```python
from build123d import *

# Parameters (mm, degrees)
SKETCH1_W                           = 17.4625
SKETCH1_H                           = 15.875
BOSS_EXTRUDE1_DEPTH                 = 9.525
SKETCH2_R                           = 4.365625
BOSS_EXTRUDE2_DEPTH                 = 4.7625
CUT_EXTRUDE1_START                  = -4.7625
CUT_EXTRUDE1_DEPTH                  = 4.7625
BOSS_EXTRUDE3_START                 = -0.0254
SKETCH4_R                           = 4.365625
BOSS_EXTRUDE3_DEPTH                 = 1.5875
CUT_EXTRUDE2_REACH                  = 28.553
CUT_EXTRUDE2_END_RADIUS             = 3
SKETCH6_W                           = 1.2375
SKETCH6_H                           = 6.35
CUT_EXTRUDE2_DIRECTION_2_REACH      = 28.553
CUT_EXTRUDE2_DIRECTION_2_END_RADIUS = 3
CHAMFER1_SIZE                       = 0.254
SKETCH7_W                           = 3.175
SKETCH7_H                           = 3.96875
BOSS_EXTRUDE4_DEPTH                 = 1.5875
BOSS_EXTRUDE5_DEPTH                 = 1.5875
FILLET1_R                           = 0.508


with BuildPart() as part:
    # Sketch1 → Boss-Extrude1 (new body)
    with BuildSketch(Plane(origin=(0, 0, 0), x_dir=(1, 0, 0), z_dir=(0, 1, 0))):
        Rectangle(SKETCH1_W, SKETCH1_H)
    extrude(amount=BOSS_EXTRUDE1_DEPTH)

    # Sketch2 → Boss-Extrude2 (add)
    with BuildSketch(Plane(origin=(0, 9.525, 0), x_dir=(1, 0, 0), z_dir=(0, 1, 0))):
        with Locations(Location((0, 0, 0), (0, 0, 90))):
            Circle(SKETCH2_R)
    extrude(amount=BOSS_EXTRUDE2_DEPTH)

    # Sketch3 → Cut-Extrude1 (cut)
    with BuildSketch(Plane(origin=(0, 14.2875, 0), x_dir=(1, 0, 0), z_dir=(0, 1, 0)).offset(CUT_EXTRUDE1_START)):
        with BuildLine():
            Line((-2.510057893, -3.571875), (2.510057893, -3.571875))
            ThreePointArc((2.510057893, -3.571875), (0, -4.365625), (-2.510057893, -3.571875))
        make_face()
        with BuildLine():
            Line((-2.510057893, 3.571875), (2.510057893, 3.571875))
            ThreePointArc((2.510057893, 3.571875), (0, 4.365625), (-2.510057893, 3.571875))
        make_face()
    extrude(amount=CUT_EXTRUDE1_DEPTH, mode=Mode.SUBTRACT)



with BuildPart() as body_2:
    # Sketch4 → Boss-Extrude3 (new body)
    with BuildSketch(Plane(origin=(0, 14.2875, 0), x_dir=(1, 0, 0), z_dir=(0, 1, 0)).offset(BOSS_EXTRUDE3_START)):
        Polygon((2.978766545, 5.159375), (-2.978766545, 5.159375), (-5.95753309, 0), (-2.978766545, -5.159375), (2.978766545, -5.159375), (5.95753309, 0), align=None)
        with Locations(Location((0, 0, 0), (0, 0, 270))):
            Circle(SKETCH4_R, mode=Mode.SUBTRACT)
    extrude(amount=-BOSS_EXTRUDE3_DEPTH)


with BuildPart() as part_1:
    add(part.part)

    add(body_2.part)  # Revolve1 merges body 2
    # Sketch5 → Revolve1 (revolve)
    with BuildSketch(Plane(origin=(0, 0, 0), x_dir=(0, 0, -1), z_dir=(1, 0, 0))):
        Polygon((-2.5, 14.2621), (-2.5, 15.2621), (-3, 15.2621), (-3, 23.7871), (0, 23.7871), (0, 14.2621), align=None)
    revolve(axis=Axis((0, 14.2621, 0), (0, -1, 0)))

    # Cut-Extrude2: up to this cylinder (the profile starts inside it)
    cut_extrude2_end = Plane(origin=(0, 20.6121, 0), z_dir=(0, 1, 0)) * Cylinder(CUT_EXTRUDE2_END_RADIUS, 64.106, mode=Mode.PRIVATE)
    # Sketch6 → Cut-Extrude2 (cut, up to the surface)
    with BuildSketch(Plane(origin=(0, 0, 0), x_dir=(0, 0, -1), z_dir=(1, 0, 0)), mode=Mode.PRIVATE) as cut_extrude2_sk1:
        with Locations((-2.38125, 20.6121)):
            Rectangle(SKETCH6_W, SKETCH6_H)
    cut_extrude2_tool1 = extrude(cut_extrude2_sk1.sketch, amount=-CUT_EXTRUDE2_REACH, mode=Mode.PRIVATE) & cut_extrude2_end
    add(cut_extrude2_tool1.solids().sort_by_distance((0, 20.6121, 2.38125))[0], mode=Mode.SUBTRACT)

    # Cut-Extrude2 direction 2: up to this cylinder (the profile starts inside it)
    cut_extrude2_direction_2_end = Plane(origin=(0, 20.6121, 0), z_dir=(0, 1, 0)) * Cylinder(CUT_EXTRUDE2_DIRECTION_2_END_RADIUS, 64.106, mode=Mode.PRIVATE)
    # Sketch6 → Cut-Extrude2 direction 2 (cut, up to the surface)
    with BuildSketch(Plane(origin=(0, 0, 0), x_dir=(0, 0, -1), z_dir=(1, 0, 0)), mode=Mode.PRIVATE) as cut_extrude2_direction_2_sk1:
        with Locations((-2.38125, 20.6121)):
            Rectangle(SKETCH6_W, SKETCH6_H)
    cut_extrude2_direction_2_tool1 = extrude(cut_extrude2_direction_2_sk1.sketch, amount=CUT_EXTRUDE2_DIRECTION_2_REACH, mode=Mode.PRIVATE) & cut_extrude2_direction_2_end
    add(cut_extrude2_direction_2_tool1.solids().sort_by_distance((0, 20.6121, 2.38125))[0], mode=Mode.SUBTRACT)

    # Chamfer1
    chamfer1_edges = [part_1.edges().sort_by_distance(p)[0] for p in [
        (0, 23.7871, -3),
    ]]
    chamfer(chamfer1_edges, length=CHAMFER1_SIZE)

    # Sketch7 → Boss-Extrude4 (add)
    with BuildSketch(Plane(origin=(0, 9.525, 0), x_dir=(1, 0, 0), z_dir=(0, 1, 0))):
        with Locations((10.31875, 0)):
            Rectangle(SKETCH7_W, SKETCH7_H)
    extrude(amount=-BOSS_EXTRUDE4_DEPTH)

    # Sketch8 → Boss-Extrude5 (add)
    with BuildSketch(Plane(origin=(0, 9.525, 0), x_dir=(1, 0, 0), z_dir=(0, 1, 0))):
        with BuildLine():
            Line((8.73125, 1.190625), (8.73125, -1.190625))
            ThreePointArc((8.73125, -1.190625), (9.921875, 0), (8.73125, 1.190625))
        make_face()
    extrude(amount=BOSS_EXTRUDE5_DEPTH)

    # Fillet1
    fillet1_edges = [part_1.edges().sort_by_distance(p)[0] for p in [
        (-8.73125, 9.525, 0),
        (0, 9.525, 7.9375),
        (8.73125, 9.525, 4.9609375),
        (0, 9.525, -7.9375),
        (8.73125, 4.7625, 7.9375),
        (-8.73125, 4.7625, 7.9375),
        (-8.73125, 4.7625, -7.9375),
        (8.73125, 4.7625, -7.9375),
        (8.73125, 9.525, -4.9609375),
        (8.73125, 8.73125, 1.984375),
        (8.73125, 8.73125, -1.984375),
        (11.90625, 8.73125, -1.984375),
        (11.90625, 8.73125, 1.984375),
        (10.31875, 9.525, 1.984375),
        (11.90625, 9.525, 0),
        (10.31875, 9.525, -1.984375),
    ]]
    fillet(fillet1_edges, radius=FILLET1_R)


solid = part_1.part
```
Work out the finished part from the listing and answer in its coordinate system (mm). A direction names the side the tool comes from. Coordinates: 2 decimals unless noted, no trailing zeros. Loops run counter-clockwise (first coordinate to the right, second up) from the corner with the lowest first, then second, coordinate; pieces in that order, holes last. Notation, with made-up numbers: M 42.25,-1 L 90.25,-1 A18 ccw 90.25,26 Z; hole C 35,28.5 d3. An arc over 180 degrees is marked long. Use CSV: the item, a comma, the result in double quotes. Start each with the question number.
(1) Given pin 1 Ø3 at (x, z) = (0.5, -0.5) entering from -Y; pin 2 Ø0.8 at (x, y) = (0, 13.5) entering from -Z; pin 3 Ø2.5 at (x, y) = (-0.5, 20.5) entering from +Z; pin 4 Ø10 at (x, y) = (2.5, 16) entering from +Z, each flat-ended and moving along its own axis, determine where each tip first touches the part or whether it passes through.
(2) Consider line 1 (Y direction, x = -3.25, z = -3.5) (3 decimals); line 2 (Y direction, x = 7.75, z = -5.75) (3 decimals); line 3 (X direction, y = 6, z = -1.75). Determine where each line is inside the solid, lowest interval first.
(3) Find section B-B, the plane z = -4.75. Give the vertices of the cut face in (x, y) (3 decimals), then the cut area to 3 significant figures.
(4) Find section D-D, the plane y = 5. Give the vertices of the cut face in (x, z).
(5) Find section A-A, the plane x = 0. State how many separate pieces and enclosed holes the cut face has, then the cut area to 3 significant figures.
(6) Find section C-C, the plane x = -7. Give the vertices of the cut face in (y, z) (1 decimal).
(7) For a pull along Z with two mould halves and no side action, classify faces 1 (the face through (11.906, 8.5, 0)), 2 (the face through (9.92, 10.31, 0.03)), 3 (the face through (0, 12, 3.572)) as +Z half, -Z half, draft (parallel to the pull), parting line (faces both ways), or undercut.
(8) For faces 4 (the face through (4.365, 11.078, 0.059)), 5 (the face through (0, 19, -3)), 6 (the face through (0, 21, 1.763)), 7 (the face through (4.49, 13.48, -2.54)), 8 (the face through (-4.447, 13.479, -2.616)), determine the directions among +Z, -Z, +X, -X, +Y, -Y from which every point of the face is accessible in a straight line to the end or side of a thin tool.
Recorded:
1,pin 1,"stops at y = 0"
1,pin 2,"stops at z = -5.16"
1,pin 3,"stops at z = 1.76"
1,pin 4,"stops at z = 5.16"
2,line 1,"y = 0 to 9.525, 12.675 to 14.262"
2,line 2,"y = 0 to 9.525"
2,line 3,"x = -8.73 to 8.73"
3,outline,"M -8.731,0 L 8.731,0 L 8.731,9.017 A0.508 ccw 8.223,9.525 L -8.223,9.525 A0.508 ccw -8.731,9.017 Z; M -3.215,12.675 L 3.215,12.675 L 3.215,14.262 L -3.215,14.262 Z"
3,area,"176 mm^2"
4,outline,"M -8.73,-7.43 A0.51 ccw -8.22,-7.94 L 8.22,-7.94 A0.51 ccw 8.73,-7.43 L 8.73,7.43 A0.51 ccw 8.22,7.94 L -8.22,7.94 A0.51 ccw -8.73,7.43 Z"
5,separate pieces,"3"
5,enclosed holes,"0"
5,area,"236 mm^2"
6,outline,"M 0,-7.9 L 9,-7.9 A0.5 ccw 9.5,-7.4 L 9.5,7.4 A0.5 ccw 9,7.9 L 0,7.9 Z"
7,face 1,"draft"
7,face 2,"parting line"
7,face 3,"undercut"
8,face 4,"none"
8,face 5,"+Y"
8,face 6,"+Z, +X, -X, +Y"
8,face 7,"-Z, +X, +Y"
8,face 8,"-Z, -X, +Y"
